from build123d import *

# Parameters (mm, degrees)
SKETCH2_W           = 35
SKETCH2_H           = 35
BOSS_EXTRUDE1_DEPTH = 800
SKETCH3_W           = 35
SKETCH3_H           = 35
BOSS_EXTRUDE2_DEPTH = 620
SKETCH5_W           = 35
SKETCH5_H           = 35
BOSS_EXTRUDE3_DEPTH = 800
SKETCH6_W           = 20
SKETCH6_H           = 690
BOSS_EXTRUDE4_DEPTH = 120
CUT_EXTRUDE1_DEPTH  = 1064.249735481


with BuildPart() as part:
    # Sketch2 → Boss-Extrude1 (new body)
    with BuildSketch(Plane(origin=(0, 0, 0), x_dir=(0, 0, -1), z_dir=(1, 0, 0))):
        with Locations((17.5, 17.5)):
            Rectangle(SKETCH2_W, SKETCH2_H)
    extrude(amount=BOSS_EXTRUDE1_DEPTH)

    # Sketch3 → Boss-Extrude2 (add)
    with BuildSketch(Plane(origin=(0, 0, -35), x_dir=(-1, 0, 0), z_dir=(0, 0, -1))):
        with Locations((-782.5, 17.5)):
            Rectangle(SKETCH3_W, SKETCH3_H)
    extrude(amount=BOSS_EXTRUDE2_DEPTH)

    # Sketch5 → Boss-Extrude3 (add)
    with BuildSketch(Plane(origin=(800, 0, 0), x_dir=(0, 0, -1), z_dir=(1, 0, 0))):
        with Locations((672.5, 17.5)):
            Rectangle(SKETCH5_W, SKETCH5_H)
    extrude(amount=-BOSS_EXTRUDE3_DEPTH)

    # Sketch6 → Boss-Extrude4 (add)
    with BuildSketch(Plane.XZ):
        with Locations((790, -345)):
            Rectangle(SKETCH6_W, SKETCH6_H)
    extrude(amount=BOSS_EXTRUDE4_DEPTH)

    # Sketch7 → Cut-Extrude1 (cut, through all)
    with BuildSketch(Plane(origin=(800, 0, 0), x_dir=(0, 0, -1), z_dir=(1, 0, 0))):
        Polygon((51.75, -80), (34.5, -120), (69, -120), align=None)
        Polygon((86.25, -80), (69, -120), (103.5, -120), align=None)
        Polygon((120.75, -80), (103.5, -120), (138, -120), align=None)
        Polygon((155.25, -80), (138, -120), (172.5, -120), align=None)
        Polygon((189.75, -80), (172.5, -120), (207, -120), align=None)
        Polygon((224.25, -80), (207, -120), (241.5, -120), align=None)
        Polygon((258.75, -80), (241.5, -120), (276, -120), align=None)
        Polygon((293.25, -80), (276, -120), (310.5, -120), align=None)
        Polygon((327.75, -80), (310.5, -120), (345, -120), align=None)
        Polygon((362.25, -80), (345, -120), (379.5, -120), align=None)
        Polygon((396.75, -80), (379.5, -120), (414, -120), align=None)
        Polygon((431.25, -80), (414, -120), (448.5, -120), align=None)
        Polygon((465.75, -80), (448.5, -120), (483, -120), align=None)
        Polygon((500.25, -80), (483, -120), (517.5, -120), align=None)
        Polygon((534.75, -80), (517.5, -120), (552, -120), align=None)
        Polygon((569.25, -80), (552, -120), (586.5, -120), align=None)
        Polygon((603.75, -80), (586.5, -120), (621, -120), align=None)
        Polygon((638.25, -80), (621, -120), (655.5, -120), align=None)
        Polygon((672.75, -80), (655.5, -120), (690, -120), align=None)
        Polygon((17.25, -80), (34.5, -120), (0, -120), align=None)
    extrude(amount=-CUT_EXTRUDE1_DEPTH, mode=Mode.SUBTRACT)


solid = part.part
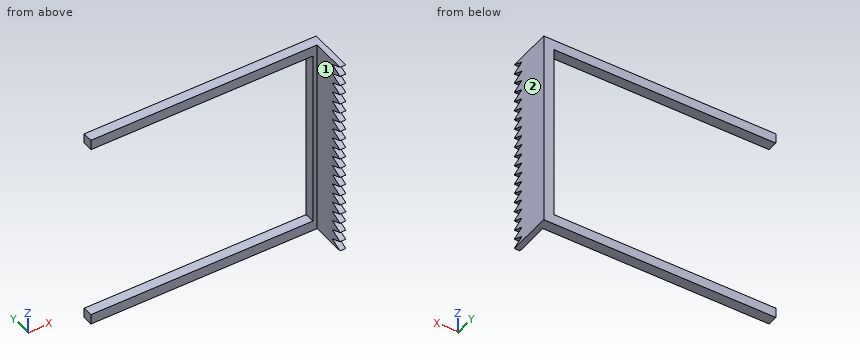
Part model, mm, in its own coordinate system. Face numbers are marked on the shaded views. A direction names the side the tool comes from. Coordinates: 2 decimals unless noted, no trailing zeros. Write each loop counter-clockwise with the first axis right and the second up, starting at its lowest first coordinate (ties: lowest second). Pieces come first, ordered by that corner, then holes. Notation, with made-up numbers: (62.25, 67.5) - (77.25, 67.5) arc R33 ccw to (77.25, 95.5) - close; hole circle Ø1 at (75, -2). An arc over 180 degrees is marked (long way). Put each result on its own line as item: value.
1. Flat gauge pin, fed straight in: pin 1 Ø6 at (y, z) = (18.5, -589.5) entering from -X. Where does the tip first touch, or does it go through?
Final values:
pin 1: stops at x = 765
2. 3-axis set-ups, long thin cutter, end or side, ignore diameter. For the marked faces 1 and 2: which of +Z, -Z, +X, -X, +Y, -Y reach the whole face in a straight line?
Final values:
face 1: +Z, -Z, -X, -Y
face 2: +Z, -Z, +X, +Y, -Y
3. Band-saw the part on B-B (y = -94). Give the number of separate pieces and of enclosed holes in the cut face, then the cut area to 3 significant figures.
Final values:
separate pieces: 21
enclosed holes: 0
area: 8,970 mm²
4. Probe line 1 along Z through (x, y) = (133, 19.5); line 2 along X through (y, z) = (-107, -443.5); line 3 along X through (y, z) = (7.5, -153.5). List the from-to ranges inside material, lowest first. Write a range as [from, to].
Final values:
line 1: z = [-690, -655], [-35, 0]
line 2: x = [780, 800]
line 3: x = [765, 800]
5. Band-saw the part on A-A (x = 653). Write the cut outline in (y, z).
Final values:
outline: (0, -690) - (35, -690) - (35, -655) - (0, -655) - close; (0, -35) - (35, -35) - (35, 0) - (0, 0) - close
